Geometry: final body of the model. Coordinates: model frame, mm. Coordinates: 2 decimals unless noted, no trailing zeros. Order: outer loops, then holes, each group sorted by start corner. A loop starts at its lowest first (then second) coordinate and runs counter-clockwise, first axis right, second up. Notation, with made-up numbers: M 31,86.5 L 89,86.5 A17 cw 89,104.5 Z; hole C -15.5,72 d9. An arc over 180 degrees is marked long. One line per question, with ' | ' between items.
from build123d import *

# Parameters (mm, degrees)
SKETCH2_R           = 105
BOSS_EXTRUDE1_DEPTH = 230
BOSS_EXTRUDE1_TAPER = 7
SKETCH3_R           = 103.5
CUT_EXTRUDE1_DEPTH  = 220
CUT_EXTRUDE1_DRAFT  = -7
CUT_EXTRUDE2_DEPTH  = 230
CUT_EXTRUDE2_DRAFT  = -7


with BuildPart() as part:
    # Sketch2 → Boss-Extrude1 (new body)
    with BuildSketch(Plane(origin=(0, 0, 0), x_dir=(1, 0, 0), z_dir=(0, 1, 0))):
        Circle(SKETCH2_R)
    extrude(amount=BOSS_EXTRUDE1_DEPTH, taper=BOSS_EXTRUDE1_TAPER)


with BuildPart() as cut_extrude1_tool:
    # Sketch3 → Cut-Extrude1 (with draft: the straight prism first)
    with BuildSketch(Plane.XZ):
        Circle(SKETCH3_R)
    extrude(amount=-CUT_EXTRUDE1_DEPTH)
    # Cut-Extrude1: the draft: its side faces are tilted about the plane it starts from
    cut_extrude1_sides = [cut_extrude1_tool.faces().sort_by_distance(p)[0] for p in [
        (-103.5, 110, 0),
    ]]
    draft(cut_extrude1_sides, Plane.XZ, CUT_EXTRUDE1_DRAFT)


with BuildPart() as part_1:
    add(part.part)

    # Cut-Extrude1: cut by cut_extrude1_tool
    add(cut_extrude1_tool.part, mode=Mode.SUBTRACT)


with BuildPart() as cut_extrude2_tool:
    # Sketch4 → Cut-Extrude2 (with draft: the straight prism first)
    with BuildSketch(Plane.XZ):
        with BuildLine():
            ThreePointArc((-105, 0), (74.246212025, -74.246212025), (0, 105))
            Line((0, 105), (0, 0))
            Line((0, 0), (-105, 0))
        make_face()
    extrude(amount=-CUT_EXTRUDE2_DEPTH)
    # Cut-Extrude2: the draft: its side faces are tilted about the plane it starts from
    cut_extrude2_sides = [cut_extrude2_tool.faces().sort_by_distance(p)[0] for p in [
        (74.246212025, 115, -74.246212025),
        (0, 115, 52.5),
        (-52.5, 115, 0),
    ]]
    draft(cut_extrude2_sides, Plane.XZ, CUT_EXTRUDE2_DRAFT)


with BuildPart() as part_2:
    add(part_1.part)

    # Cut-Extrude2: cut by cut_extrude2_tool
    add(cut_extrude2_tool.part, mode=Mode.SUBTRACT)


solid = part_2.part
1. Section A-A, the plane y = 24.5. Output: boundary loops of the cut face in (x, z).
Response values:
outline: M -101.95,-3.01 L -100.45,-3.01 A100.49 cw 3.01,100.45 L 3.01,101.95 A101.99 ccw Z
2. Pin query (flat end, axial travel): P1, Ø2, axis at y = 123.5, z = 54, coming from the +X side; P2, Ø1.5, axis at y = 27.5, z = 37.5, coming from the -X side; P3, Ø6, axis at x = -73.5, y = 166, coming from the -Z side. Return the tip coordinate at first contact, or that it passes through.
Response values:
P1: stops at x = -69.11 | P2: stops at x = -94.76 | P3: stops at z = 32.44
3. Draft query along Z for faces 1 (the face through (-79.967, 0, 67.811)), 2 (the face through (-62.74, 108.46, 64.78)), 3 (the face through (-38.07, 225.2, -27.65)). Return one class per face: pulls with the +Z half, pulls with the -Z half, needs draft (parallel to the pull), parting line crosses it, or undercut.
Response values:
face 1: needs draft | face 2: undercut | face 3: pulls with the -Z half
4. Section B-B, the plane y = 124.5. Output: boundary loops of the cut face in (x, z), and give its area (3 significant figures).
Response values:
outline: M -88.4,-15.29 L -86.88,-15.29 A88.21 cw 15.29,86.88 L 15.29,88.4 A89.71 ccw Z | area: 256 mm^2
5. Material intervals for line 1 (Y direction, x = -42, z = 57); line 2 (Z direction, x = 1, y = 138); line 3 (Z direction, x = -39.5, y = 204), sorted ascending. Write a range as [from, to].
Response values:
line 1: y = [220, 230] | line 2: z = [86.55, 88.05] | line 3: z = [67.78, 69.51]
